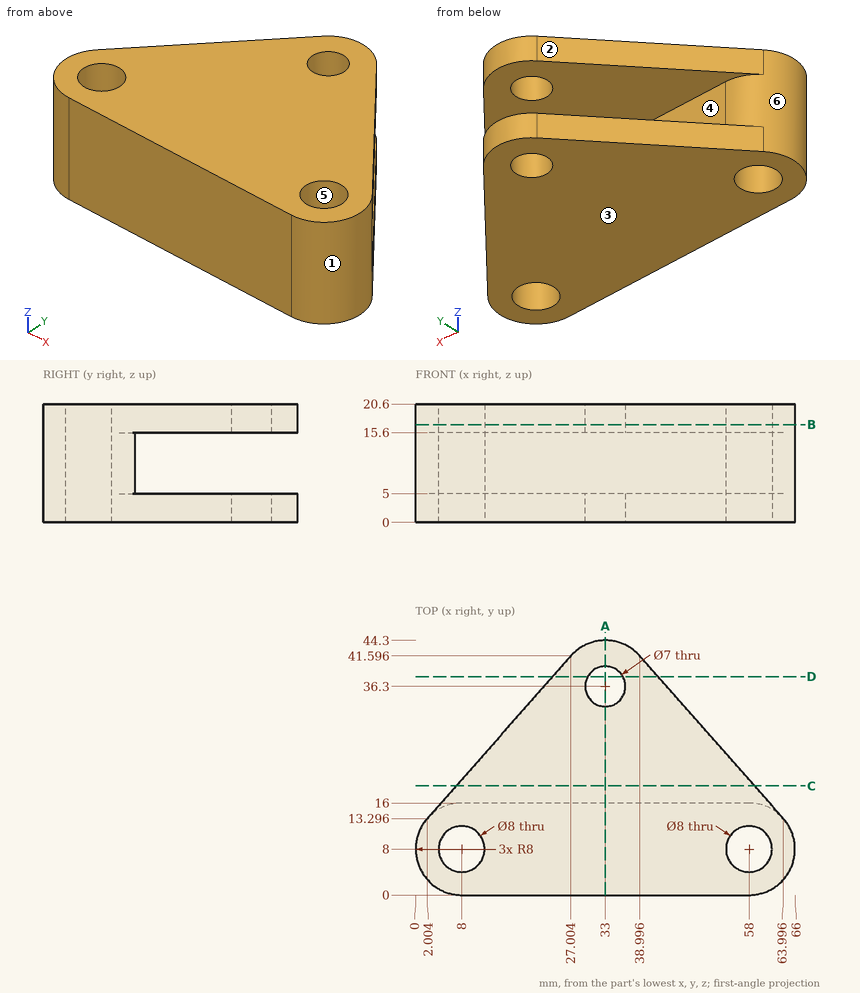
Can you work these out from the drawing? Everything is in mm from the part's minimum corner. A direction names the side the tool comes from. Give positions to 0.01 mm unless a question says otherwise; leave off trailing zeros. Order: outer loops, then holes, each group sorted by start corner. A loop starts at its lowest first (then second) coordinate and runs counter-clockwise, first axis right, second up. Notation, with made-up numbers: M 27.25,88 L 80.25,88 A18 cw 80.25,97 Z; hole C 0.5,-16 d6. An arc over 180 degrees is marked long. One line per question, with ' | ' between items.
1. We'd pull the mould along Z, two halves only. Please class the marked faces 1, 2 and 3: +Z half, -Z half, draft (parallel to the pull), parting line (faces both ways), or undercut.
Results:
face 1: undercut | face 2: draft | face 3: -Z half
2. I want a section at C-C (y = 19). List the corners of the cut face in (x, z) for me.
Results:
outline: M 7.04,0 L 58.96,0 L 58.96,5 L 7.04,5 Z; M 7.04,15.6 L 58.96,15.6 L 58.96,20.6 L 7.04,20.6 Z
3. I'm going to push flat-ended pins straight in: pin 1 (2 mm diameter, centred on x = 10, z = 10, fed in from +Y); pin 2 (6.5 mm diameter, centred on x = 58, y = 8, fed in from +Z); pin 3 (1 mm diameter, centred on y = 11.5, z = 6, fed in from -X); pin 4 (4 mm diameter, centred on x = 24, z = 14, fed in from +Y) (1 decimal). Where does each tip first touch, or does it pass through?
Results:
pin 1: y = 16 | pin 2: through | pin 3: x = 0.58 | pin 4: y = 39.6
4. For the marked faces 4, 5 and 6, which set-ups out of +Z, -Z, +X, -X, +Y, -Y let a thin tool reach every point of the face, with its end or its side?
Results:
face 4: +X, -X, +Y | face 5: +Z, -Z | face 6: -X
5. I want a section at B-B (z = 17). List the corners of the cut face in (x, y) for me (1 decimal).
Results:
outline: M 2,13.3 A8 ccw 8,0 L 58,0 A8 ccw 64,13.3 L 39,41.6 A8 ccw 27,41.6 Z; hole C 8,8 d8; hole C 33,36.3 d7; hole C 58,8 d8
6. I want a section at A-A (x = 33). List the corners of the cut face in (y, z) for me.
Results:
outline: M 0,0 L 32.8,0 L 32.8,5 L 16,5 L 16,15.6 L 32.8,15.6 L 32.8,20.6 L 0,20.6 Z; M 39.8,0 L 44.3,0 L 44.3,5 L 39.8,5 Z; M 39.8,15.6 L 44.3,15.6 L 44.3,20.6 L 39.8,20.6 Z
7. I want a section at D-D (y = 38). List the corners of the cut face in (x, z) for me, and give its area (3 significant figures).
Results:
outline: M 23.83,0 L 29.94,0 L 29.94,5 L 23.83,5 Z; M 23.83,15.6 L 29.94,15.6 L 29.94,20.6 L 23.83,20.6 Z; M 36.06,0 L 42.17,0 L 42.17,5 L 36.06,5 Z; M 36.06,15.6 L 42.17,15.6 L 42.17,20.6 L 36.06,20.6 Z | area: 122 mm²
8. If I drill on line 1 (Y direction, x = 33, z = 17.05); line 2 (Z direction, x = 40, y = 22.5); line 3 (X direction, y = 10.5, z = 18.75), over which ranges is the centre line in solid material (lowest first)?
Results:
line 1: 0 to 32.8, 39.8 to 44.3 | line 2: 0 to 5, 15.6 to 20.6 | line 3: 0.4 to 4.88, 11.12 to 54.88, 61.12 to 65.6
